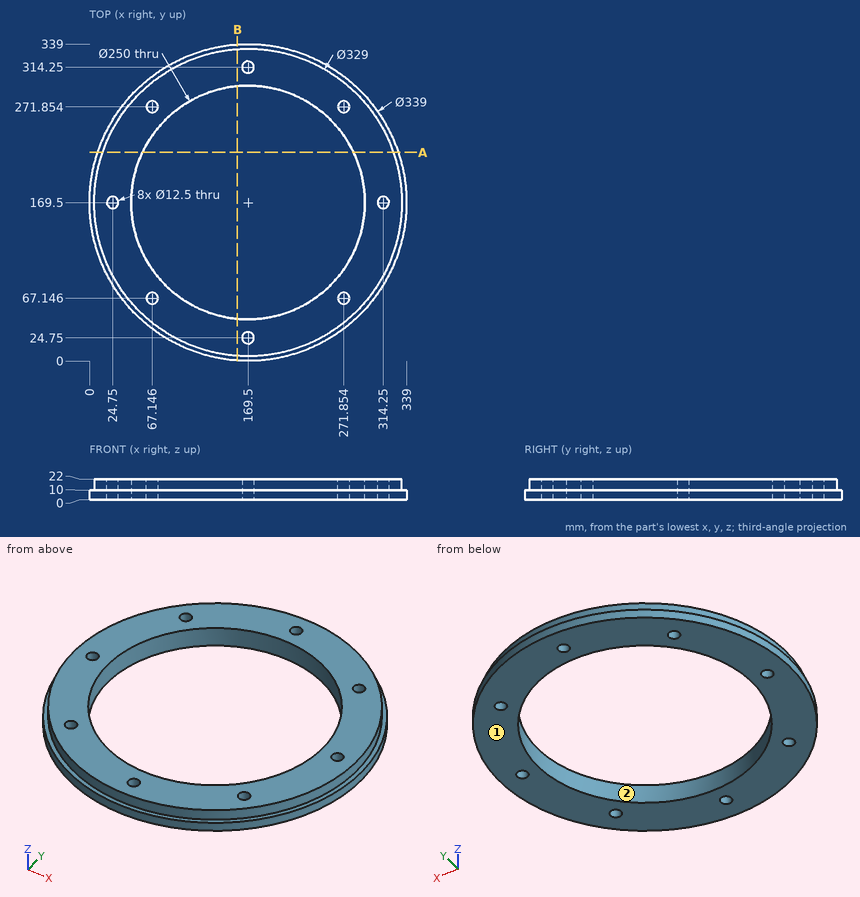
Drawing for the job (mm, zero at the part's lowest x, y, z). Give positions to 0.01 mm unless a question says otherwise; leave off trailing zeros. Loops run counter-clockwise (first coordinate to the right, second up) from the corner with the lowest first, then second, coordinate; pieces in that order, holes last.
1) Band-saw the part on B-B on x = 158. List the corners of the cut face in (y, z).
Values follow:
outline: (0.39, 0) - (45.03, 0) - (45.03, 22) - (5.4, 22) - (5.4, 10) - (0.39, 10) - close; (293.97, 0) - (338.61, 0) - (338.61, 10) - (333.6, 10) - (333.6, 22) - (293.97, 22) - close
2) Band-saw the part on A-A on y = 223. List the corners of the cut face in (x, z) (1 decimal).
Values follow:
outline: (8.7, 0) - (56.5, 0) - (56.5, 22) - (13.9, 22) - (13.9, 10) - (8.7, 10) - close; (282.5, 0) - (330.3, 0) - (330.3, 10) - (325.1, 10) - (325.1, 22) - (282.5, 22) - close
3) Drop flat-ended pins along their axis: P1, Ø2, axis at x = 82, z = 3, coming from the +Y side; P2, Ø4, axis at y = 180, z = 18, coming from the -X side; P3, Ø4, axis at x = 276.5, y = 266, coming from the -Z side; P4, Ø5, axis at x = 257.5, z = 14, coming from the -Y side (1 decimal). Give the stop position or say it passes through.
Values follow:
P1: stops at y = 315.27
P2: stops at x = 5.22
P3: stops at z = 0
P4: stops at y = 29
4) Probe line 1 along Y through (x, z) = (65.5, 10.25) (1 decimal); line 2 along Y through (x, z) = (98, 16.25); line 3 along X through (y, z) = (141, 5.5). List the from-to ranges inside material, lowest first.
Values follow:
line 1: y = 42 to 61.1, 73.2 to 100.2, 238.8 to 265.8, 277.9 to 297
line 2: y = 21.35 to 66.97, 272.03 to 317.65
line 3: x = 2.41 to 47.79, 291.21 to 336.59
5) Two-plate mould, pull along Y, no slides. Class the marked faces 1 and 2: released by +Y, released by -Y, zero draft, split by the parting line, or undercut.
Values follow:
face 1: zero draft
face 2: undercut
